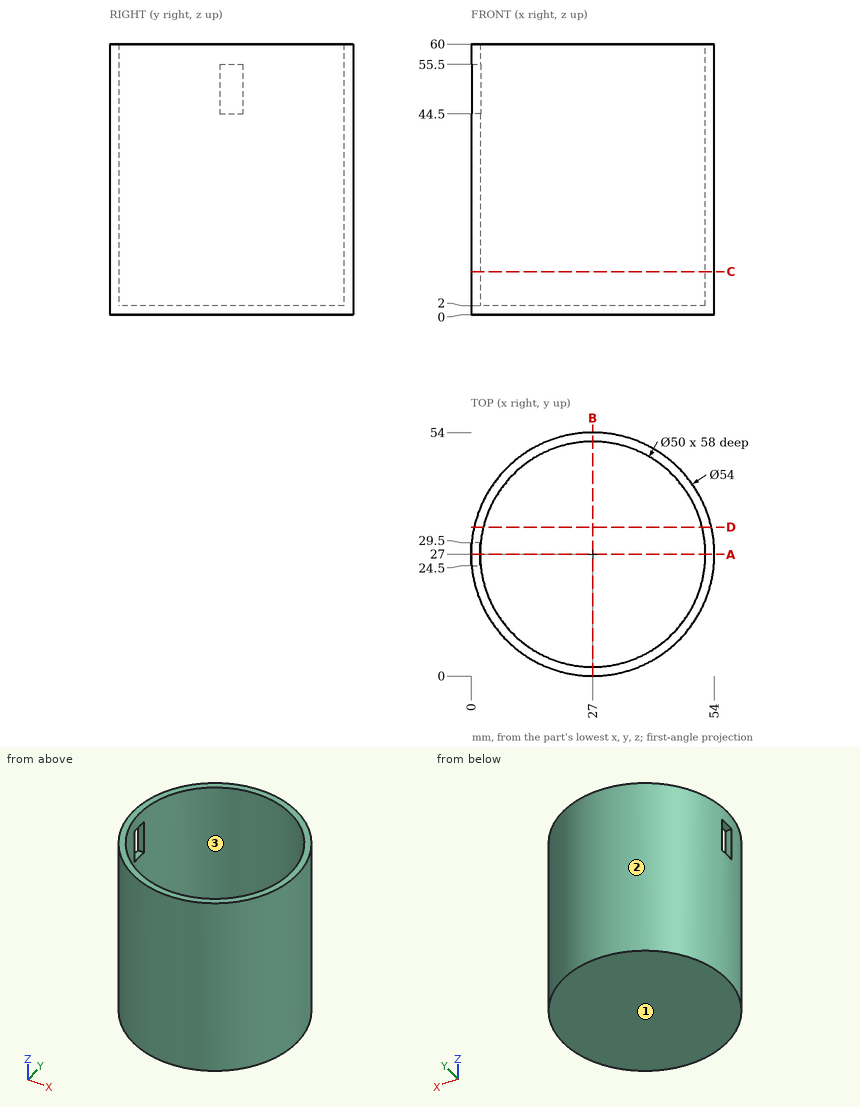
Answer from the drawing. Dimensions are ordinates in mm from the lowest x, y and z of the part. Give positions to 0.01 mm unless a question says otherwise; leave off trailing zeros. Order: outer loops, then holes, each group sorted by start corner. A loop starts at its lowest first (then second) coordinate and runs counter-clockwise, first axis right, second up. Notation, with made-up numbers: (-22.75, -16.5) - (28.25, -16.5) arc R14 ccw to (28.25, 8.5) - close; hole circle Ø7 at (85.25, -17). An arc over 180 degrees is marked (long way). One line per item, written item: value. Start each with the question number.
1. Section D-D, the plane y = 33 is taken. Write down the section's boundary in (x, z).
2. Section A-A, the plane y = 27 is taken. Write down the section's boundary in (x, z), then the cut area to 3 significant figures.
3. Consider line 1 (Y direction, x = 27, z = 46); line 2 (Z direction, x = 26.5, y = 45). Determine where each line is inside the solid, lowest interval first.
4. Each of these flat-tipped pins is pushed along its axis until it touches: pin 1 Ø8 at (x, y) = (38.5, 15) entering from +Z; pin 2 Ø2 at (y, z) = (17, 28.5) entering from -X; pin 3 Ø1.6 at (x, z) = (1.5, 52.5) entering from +Y. Where does it stop, or does it pass through?
5. Section C-C, the plane z = 9.5 is taken. Write down the section's boundary in (x, y), then the cut area to 3 significant figures.
6. For a pull along Y with two mould halves and no side action, classify the marked faces 1, 2 and 3 as released by +Y, released by -Y, zero draft, split by the parting line, or undercut.
7. Section B-B, the plane x = 27 is taken. Write down the section's boundary in (y, z).
Filled sheet:
1. outline: (0.68, 0) - (53.32, 0) - (53.32, 60) - (51.27, 60) - (51.27, 2) - (2.73, 2) - (2.73, 60) - (0.68, 60) - close
2. outline: (0, 0) - (54, 0) - (54, 60) - (52, 60) - (52, 2) - (2, 2) - (2, 44.5) - (0, 44.5) - close; (0, 55.5) - (2, 55.5) - (2, 60) - (0, 60) - close
2. area: 318 mm²
3. line 1: 0 to 2, 52 to 54
3. line 2: 0 to 2
4. pin 1: z = 2
4. pin 2: x = 1.54
4. pin 3: y = 37.9
5. outline: circle Ø54 at (27, 27); hole circle Ø50 at (27, 27)
5. area: 327 mm²
6. face 1: zero draft
6. face 2: split by the parting line
6. face 3: undercut
7. outline: (0, 0) - (54, 0) - (54, 60) - (52, 60) - (52, 2) - (2, 2) - (2, 60) - (0, 60) - close
